```python
from build123d import *

# Parameters (mm, degrees)
IZIM10_W                    = 180
IZIM10_H                    = 180
Y_KSEKLIK_EKSTR_ZYON1_DEPTH = 108
KES_EKSTR_ZYON7_DEPTH       = 108
IZIM13_R                    = 115.75
Y_KSEKLIK_EKSTR_ZYON2_DEPTH = 550
IZIM14_R                    = 109.75
KES_EKSTR_ZYON8_DEPTH       = 294
IZIM15_W                    = 180
IZIM15_H                    = 96
KES_EKSTR_ZYON9_DEPTH       = 294
IZIM16_R                    = 5
KES_EKSTR_ZYON10_DEPTH      = 294


with BuildPart() as part:
    # Çizim10 → Yükseklik-Ekstrüzyon1 (new body)
    with BuildSketch(Plane.XY):
        with Locations((90, 90)):
            Rectangle(IZIM10_W, IZIM10_H)
    extrude(amount=Y_KSEKLIK_EKSTR_ZYON1_DEPTH)

    # Çizim11 → Kes-Ekstrüzyon7 (cut)
    with BuildSketch(Plane.XY.offset(108)):
        with BuildLine():
            ThreePointArc((0, 90), (26.360389693, 153.639610307), (90, 180))
            Line((90, 180), (0, 180))
            Line((0, 180), (0, 90))
        make_face()
        with BuildLine():
            ThreePointArc((90, 0), (26.360389693, 26.360389693), (0, 90))
            Line((0, 90), (0, 0))
            Line((0, 0), (90, 0))
        make_face()
    extrude(amount=-KES_EKSTR_ZYON7_DEPTH, mode=Mode.SUBTRACT)

    # Çizim13 → Yükseklik-Ekstrüzyon2 (add)
    with BuildSketch(Plane(origin=(180, 0, 0), x_dir=(0, 0, -1), z_dir=(1, 0, 0))):
        with Locations((-54, 90)):
            Circle(IZIM13_R)
    extrude(amount=Y_KSEKLIK_EKSTR_ZYON2_DEPTH)

    # Çizim14 → Kes-Ekstrüzyon8 (cut)
    with BuildSketch(Plane(origin=(730, 0, 0), x_dir=(0, 0, -1), z_dir=(1, 0, 0))):
        with Locations((-54, 90)):
            Circle(IZIM14_R)
    extrude(amount=-KES_EKSTR_ZYON8_DEPTH, mode=Mode.SUBTRACT)

    # Çizim15 → Kes-Ekstrüzyon9 (cut)
    with BuildSketch(Plane(origin=(0, 180, 0), x_dir=(1, 0, 0), z_dir=(0, 1, 0))):
        with Locations((90, -54)):
            Rectangle(IZIM15_W, IZIM15_H)
    extrude(amount=-KES_EKSTR_ZYON9_DEPTH, mode=Mode.SUBTRACT)

    # Çizim16 → Kes-Ekstrüzyon10 (cut)
    with BuildSketch(Plane.XY.offset(108)):
        with Locations((90, 90)):
            Circle(IZIM16_R)
    extrude(amount=-KES_EKSTR_ZYON10_DEPTH, mode=Mode.SUBTRACT)


solid = part.part
```
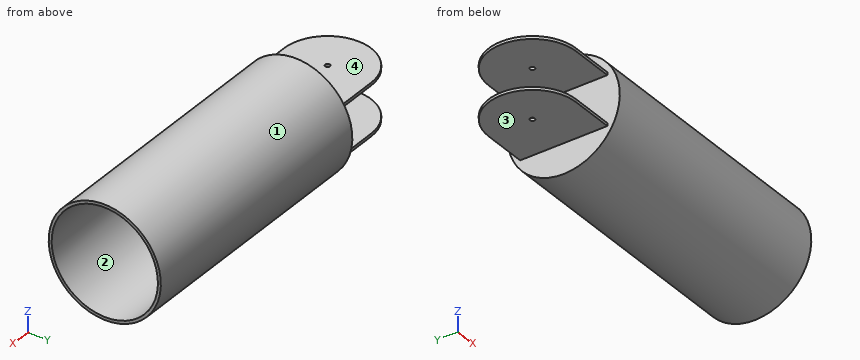
Verification items for the finished model (mm, model axes). Face numbers are marked on the shaded views. Coordinates: 2 decimals unless noted, no trailing zeros. Write each loop counter-clockwise with the first axis right and the second up, starting at its lowest first coordinate (ties: lowest second). Pieces come first, ordered by that corner, then holes. Notation, with made-up numbers: M 89,59 L 138,59 A33 cw 138,95 Z; hole C 46,85 d3. An arc over 180 degrees is marked long. Answer as a JSON object with one key per item and string values. Group by question number.
(1) Material ranges on line 1 (Y direction, x = 478, z = 54); line 2 (Y direction, x = 90, z = 2); line 3 (Z direction, x = 163, y = 171), recorded low to high.
(2) Gauge pin test, flat ends, axial feed: pin 1 (5 mm diameter, centred on x = 314.5, z = 11, fed in from -Y); pin 2 (1.8 mm diameter, centred on x = 122.5, z = 105, fed in from -Y); pin 3 (12 mm diameter, centred on y = 42, z = -23.5, fed in from -X). Record the tip position at first contact, or that the pin passes through.
(3) Cross-section at C-C, the plane y = 127. Record the cut outline in (x, z), and give its area (3 significant figures).
(4) Cross-section at D-D, the plane x = 333. Record the cut outline in (y, z).
(5) Release check for a two-part mould opening along Z. For the marked faces 1, 2, 3 and 4 record: +Z half, -Z half, draft (parallel to the pull), parting line (faces both ways), or undercut.
(6) Cross-section at B-B, the plane x = 487. Record the cut outline in (y, z).
(7) Cross-section at A-A, the plane z = 54. Record the cut outline in (x, y), and give its area (3 significant figures).
Reply:
{
 "1": {"line 1": "-25.75 to -19.75, 199.75 to 205.75", "line 2": "0 to 85, 95 to 180", "line 3": "0 to 6, 102 to 108"},
 "2": {"pin 1": "y = -18.43", "pin 2": "y = 0", "pin 3": "x = 180"},
 "3": {"outline": "M 7.96,0 L 180,0 L 180,-55.68 L 730,-55.68 L 730,-49.33 L 436,-49.33 L 436,157.33 L 730,157.33 L 730,163.68 L 180,163.68 L 180,108 L 7.96,108 L 7.96,102 L 180,102 L 180,6 L 7.96,6 Z", "area": "62,000 mm²"},
 "4": {"outline": "C 90,54 d231.5"},
 "5": {"face 1": "parting line", "face 2": "undercut", "face 3": "-Z half", "face 4": "+Z half"},
 "6": {"outline": "C 90,54 d231.5; hole C 90,54 d219.5"},
 "7": {"outline": "M 180,-25.75 L 730,-25.75 L 730,-19.75 L 436,-19.75 L 436,199.75 L 730,199.75 L 730,205.75 L 180,205.75 Z", "area": "62,800 mm²"}
}
